```python
from build123d import *

# Parameters (mm, degrees)
BOSS_EXTRUDE1_DEPTH = 42


with BuildPart() as part:
    # Sketch1 → Boss-Extrude1 (new body)
    with BuildSketch(Plane(origin=(0, 0, 0), x_dir=(1, 0, 0), z_dir=(0, 1, 0))):
        with BuildLine():
            Line((-58.112270696, -119.940697821), (-51.585786438, -113.414213562))
            ThreePointArc((-51.585786438, -113.414213562), (-51.152240935, -112.765366865), (-51, -112))
            Line((-51, -112), (-51, -104))
            Line((-51, -104), (-50, -104))
            Line((-50, -104), (-50, -112))
            ThreePointArc((-50, -112), (-50.228361402, -113.148050297), (-50.878679656, -114.121320344))
            Line((-50.878679656, -114.121320344), (-57.405163915, -120.647804602))
            ThreePointArc((-57.405163915, -120.647804602), (-58.508770183, -124.210475144), (-56.193825287, -127.134786741))
            ThreePointArc((-56.193825287, -127.134786741), (0, -139), (56.193825287, -127.134786741))
            ThreePointArc((56.193825287, -127.134786741), (58.508770183, -124.210475144), (57.405163915, -120.647804602))
            Line((57.405163915, -120.647804602), (50.878679656, -114.121320344))
            ThreePointArc((50.878679656, -114.121320344), (50.228361402, -113.148050297), (50, -112))
            Line((50, -112), (50, -104))
            Line((50, -104), (51, -104))
            Line((51, -104), (51, -112))
            ThreePointArc((51, -112), (51.152240935, -112.765366865), (51.585786438, -113.414213562))
            Line((51.585786438, -113.414213562), (58.112270696, -119.940697821))
            ThreePointArc((58.112270696, -119.940697821), (59.491778531, -124.394035998), (56.598097412, -128.049425494))
            ThreePointArc((56.598097412, -128.049425494), (0, -140), (-56.598097412, -128.049425494))
            ThreePointArc((-56.598097412, -128.049425494), (-59.491778531, -124.394035998), (-58.112270696, -119.940697821))
        make_face()
    extrude(amount=BOSS_EXTRUDE1_DEPTH)


solid = part.part
```
Could you check a few things on this model? Use its own coordinates, in mm. A direction names the side the tool comes from. Coordinates: 2 decimals unless noted, no trailing zeros. Order: outer loops, then holes, each group sorted by start corner. A loop starts at its lowest first (then second) coordinate and runs counter-clockwise, first axis right, second up. Notation, with made-up numbers: M -29.75,67.5 L -10.75,67.5 A7 ccw -10.75,71.5 Z; hole C -6,13.25 d9. An arc over 180 degrees is marked long. Use one line per item in the form item = value. Start each with the question number.
1. Suppose I cut it at A-A on z = 107. Write out the boundary of the cut face in (x, y), then the cut area to 3 significant figures.
2. Suppose I cut it at B-B on y = 34. Write out the boundary of the cut face in (x, z).
3. We'd pull the mould along X, two halves only. Please class faces 4 (the cylindrical face through (-59.48, 20.71, 124.46)), 5 (the flat face through (0.3, 42, 139.2)), 6 (the flat face through (-50, 21, 108)): +X half, -X half, draft (parallel to the pull), parting line (faces both ways), or undercut.
4. Please list where these lines run through material, in increasing order: line 1 (X direction, y = 19, z = 109); line 2 (X direction, y = 13, z = 128); line 3 (Z direction, x = -53, y = 26.5).
5. Suppose I cut it at C-C on z = 132.5. Write out the boundary of the cut face in (x, y).
6. On a 3-axis mill with a long thin cutter (end or side, diameter ignored), from which of +Z, -Z, +X, -X, +Y, -Y can I reach the whole of each face in a straight line? I mean faces 1 (the flat face through (51, 21, 108)), 2 (the flat face through (-51, 21, 108)), 3 (the flat face through (54.19, 20.71, 117.43)). Say none if no direction works.
7. Suppose I cut it at D-D on x = -22. Write out the boundary of the cut face in (y, z).
8. For pin 1 (4 mm diameter, centred on y = 30.5, z = 107, fed in from -X); pin 2 (9 mm diameter, centred on y = 19.5, z = 109, fed in from -X); pin 3 (2.5 mm diameter, centred on y = 10.5, z = 108.5, fed in from +X); pin 4 (10 mm diameter, centred on x = -19.5, z = 128, fed in from +Y), each with a flat end and sliding along its axis, tell me the tip position at first contact or that it passes through.
Geometry says:
q1.outline = M -51,0 L -50,0 L -50,42 L -51,42 Z; M 50,0 L 51,0 L 51,42 L 50,42 Z
q1.area = 84.0 mm^2
q2.outline = M -58.11,119.94 L -51.59,113.41 A2 cw -51,112 L -51,104 L -50,104 L -50,112 A3 ccw -50.88,114.12 L -57.41,120.65 A4 cw -56.19,127.13 A139 cw 56.19,127.13 A4 cw 57.41,120.65 L 50.88,114.12 A3 ccw 50,112 L 50,104 L 51,104 L 51,112 A2 cw 51.59,113.41 L 58.11,119.94 A5 ccw 56.6,128.05 A140 ccw -56.6,128.05 A5 ccw Z
q3.face_4 = -X half
q3.face_5 = draft
q3.face_6 = undercut
q4.line_1 = -51 to -50, 50 to 51
q4.line_2 = -56.71 to -54.19, 54.19 to 56.71
q4.line_3 = 114.83 to 116.24, 128.5 to 129.58
q5.outline = M -45.21,0 L -42.01,0 L -42.01,42 L -45.21,42 Z; M 42.01,0 L 45.21,0 L 45.21,42 L 42.01,42 Z
q6.face_1 = -Z, +X, +Y, -Y
q6.face_2 = -Z, -X, +Y, -Y
q6.face_3 = +Y, -Y
q7.outline = M 0,137.25 L 42,137.25 L 42,138.26 L 0,138.26 Z
q8.pin_1 = -51
q8.pin_2 = -51.67
q8.pin_3 = 51
q8.pin_4 = through
